Read the model definition and answer for the solid it produces. Units are mm, in the model's axes. Face numbers are marked on the shaded views. A direction names the side the tool comes from. Coordinates: 2 decimals unless noted, no trailing zeros. Write each loop counter-clockwise with the first axis right and the second up, starting at its lowest first coordinate (ties: lowest second). Pieces come first, ordered by that corner, then holes. Notation, with made-up numbers: (18, 50.5) -> (24, 50.5) arc R17 cw to (24, 55.5) -> close; hole circle Ø1 at (18, -14). An arc over 180 degrees is marked (long way). One line per item, written item: value. Start each with the question number.
1. Given P1, Ø2, axis at y = -40.5, z = -4.5, coming from the +X side; P2, Ø2, axis at y = -28.5, z = -2, coming from the -X side; P3, Ø1, axis at x = 23, z = -4, coming from the +Y side, each flat-ended and moving along its own axis, determine where each tip first touches the part or whether it passes through.
2. For the marked faces 1 and 2, determine the directions among +Z, -Z, +X, -X, +Y, -Y from which every point of the face is accessible in a straight line to the end or side of a thin tool.
3. Find section A-A, the plane y = -40. Write down the section's boundary in (x, z), and give its area (3 significant figures).
4. Find section B-B, the plane x = 31. Write down the section's boundary in (y, z).
5. Consider line 1 along Y through (x, z) = (39.5, -3.25); line 2 along Z through (x, y) = (43, -73.5); line 3 along X through (y, z) = (-37, -1.25). Determine where each line is inside the solid, lowest interval first.
6. Find section D-D, the plane y = -24. Write down the section's boundary in (x, z), and give its area (3 significant figures).
7. Find section C-C, the plane z = -5.25. Write down the section's boundary in (x, y), and give its area (3 significant figures).
Autodesk Inventor part; units mm, degrees
ref_plane "YZ Plane" through (0, 0, 0) normal (1, 0, 0) x (0, 1, 0)
ref_plane "XZ Plane" through (0, 0, 0) normal (0, 1, 0) x (-1, 0, 0)
ref_plane "XY Plane" through (0, 0, 0) normal (0, 0, 1) x (1, 0, 0)
sketch "스케치1" plane through (0, 0, 0) normal (0, 0, 1) x (1, 0, 0)
  line L0 (0, 0) -> (80, 0)
  line L1 (80, 0) -> (80, -80)
  line L2 (80, -80) -> (0, -80)
  line L3 (0, -80) -> (0, 0)
  dimension "d0" = 80
  dimension "d1" = 80
extrude "돌출1" add sketch "스케치1" along normal blind 1
sketch "스케치2" plane through (0, 0, 0) normal (0, 0, -1) x (-1, 0, 0)
  circle A0 centre (-40, -40) radius 15
  point P0 (0, 0)
  dimension "d4" = 40
  dimension "d5" = 40
  dimension "d6" = 30
extrude "돌출2" add sketch "스케치2" along normal blind 10
properties part number "배경"
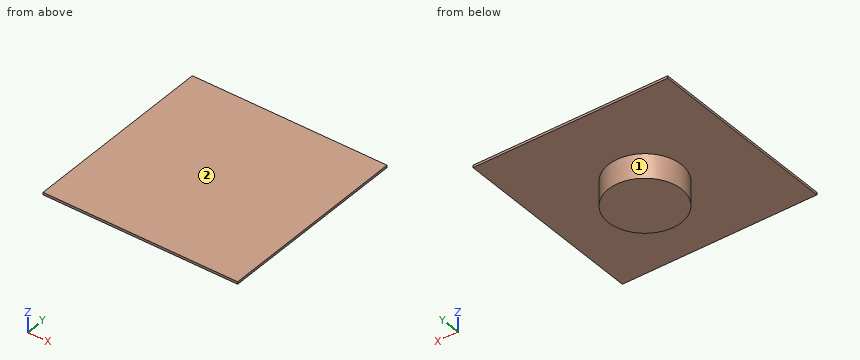
Answer block:
1. P1: stops at x = 55
1. P2: stops at x = 29.29
1. P3: passes through
2. face 1: -Z
2. face 2: +Z, +X, -X, +Y, -Y
3. outline: (0, 0) -> (25, 0) -> (25, -10) -> (55, -10) -> (55, 0) -> (80, 0) -> (80, 1) -> (0, 1) -> close
3. area: 380 mm2
4. outline: (-80, 0) -> (-52, 0) -> (-52, -10) -> (-28, -10) -> (-28, 0) -> (0, 0) -> (0, 1) -> (-80, 1) -> close
5. line 1: y = -54.99 to -25.01
5. line 2: z = 0 to 1
5. line 3: x = 25.3 to 54.7
6. outline: (0, 0) -> (80, 0) -> (80, 1) -> (0, 1) -> close
6. area: 80.0 mm2
7. outline: circle Ø30 at (40, -40)
7. area: 707 mm2
